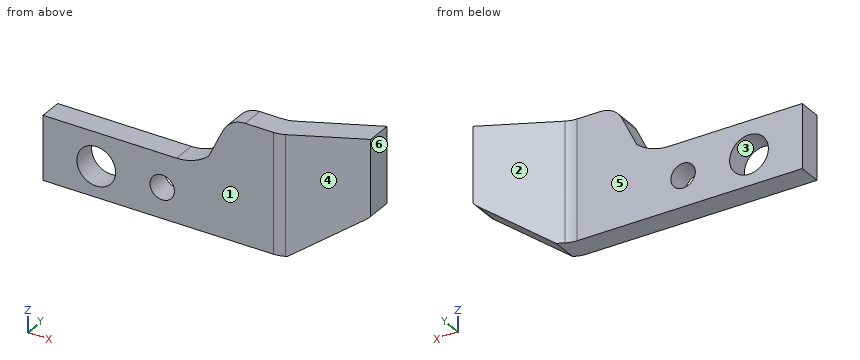
from build123d import *

# Parameters (mm, degrees)
SALIENTE_EXTRUIR1_DEPTH    = 100
CORTAR_EXTRUIR3_START      = -9.53
CORTAR_EXTRUIR3_DEPTH      = 27.53
CORTAR_EXTRUIR4_DEPTH      = 217.130875219
CORTAR_EXTRUIR4_DEPTH_BACK = 217.130875219
CROQUIS5_R                 = 6
CORTAR_EXTRUIR5_DEPTH      = 216.124741308
CORTAR_EXTRUIR5_DEPTH_BACK = 216.124741308
CROQUIS6_R                 = 5
SALIENTE_EXTRUIR5_START    = 15.13
CROQUIS12_R                = 8
CROQUIS12_R_2              = 6
SALIENTE_EXTRUIR5_DEPTH    = 15.13
CROQUIS14_R                = 10
CROQUIS14_R_2              = 6
SALIENTE_EXTRUIR6_DEPTH    = 14.13
REDONDEO1_R                = 10
CROQUIS15_R                = 129.913958972
CORTAR_EXTRUIR6_DEPTH      = 241.731126452
CORTAR_EXTRUIR7_DEPTH      = 241.731126452
CORTAR_EXTRUIR7_DEPTH_BACK = 241.731126452
CROQUIS16_R                = 167.818918699
CROQUIS16_W                = 152.833455663
CROQUIS16_H                = 57.32474986
CROQUIS17_R                = 7.94
CORTAR_EXTRUIR8_DEPTH      = 275.18730081


# Read off the part's stored shape, not the designer's step: Cortar-Extruir3
with BuildPart() as part:
    # Croquis1 → Saliente-Extruir1 (new body)
    with BuildSketch(Plane(origin=(0, 0, 0), x_dir=(-1, 0, 0), z_dir=(0, 0, 1))):
        Polygon((197, -18), (95.487511072, -18), (58.434265153, 0), (0, 0), (0, -9.53), (56.241982635, -9.53), (93.295228555, -27.53), (197, -27.53), align=None)
    extrude(amount=SALIENTE_EXTRUIR1_DEPTH)

    # Cortar-Extruir3 outline → Cortar-Extruir3 (cut)
    with BuildSketch(Plane.XZ.offset(-18).offset(CORTAR_EXTRUIR3_START)):
        with BuildLine():
            ThreePointArc((-55.249840127, 84.500440573), (-26.332291795, 96.782267833), (-21.152892526, 65.794500802))
            Line((-21.152892526, 65.794500802), (-64.625951049, 17.972279409))
            ThreePointArc((-64.625951049, 17.972279409), (-65.478127712, 17.140282818), (-66.423173576, 16.415498915))
            Line((-66.423173576, 16.415498915), (-90.606375863, 0.05961622))
            ThreePointArc((-90.606375863, 0.05961622), (-90.650882543, 0.029688544), (-90.695549093, 0))
            Line((-90.695549093, 0), (0, 0))
            Line((0, 0), (0, 100))
            Line((0, 100), (-197, 100))
            Line((-197, 100), (-197, 0))
            Line((-197, 0), (-190.011984345, 0))
            Line((-190.011984345, 0), (-190.011984345, 26.126101457))
            Line((-190.011984345, 26.126101457), (-135.299104154, 26.091319242))
            ThreePointArc((-135.299104154, 26.091319242), (-128.302319283, 27.350377114), (-122.187975643, 30.977363067))
            Line((-122.187975643, 30.977363067), (-116.240808663, 43.251828603))
            ThreePointArc((-116.240808663, 43.251828603), (-112.551713447, 47.365099857), (-107.241491018, 48.891521053))
            Line((-107.241491018, 48.891521053), (-89.308606426, 48.891521053))
            ThreePointArc((-89.308606426, 48.891521053), (-87.268864218, 49.101758455), (-85.31488803, 49.723630708))
            ThreePointArc((-85.31488803, 49.723630708), (-66.329070141, 63.694356674), (-55.249840127, 84.500440573))
        make_face()
    extrude(amount=CORTAR_EXTRUIR3_DEPTH, mode=Mode.SUBTRACT)

    # Croquis5 → Cortar-Extruir4 (cut, two sides: drawn at the far end of the back side and taken through both)
    with BuildSketch(Plane.XZ.offset(-CORTAR_EXTRUIR4_DEPTH_BACK)):
        with Locations(Location((-35.951954024, 79.247670643, 0), (0, 0, 270))):
            Circle(CROQUIS5_R)
    extrude(amount=CORTAR_EXTRUIR4_DEPTH + CORTAR_EXTRUIR4_DEPTH_BACK, mode=Mode.SUBTRACT)

    # Croquis6 → Cortar-Extruir5 (cut, two sides: drawn at the far end of the back side and taken through both)
    with BuildSketch(Plane.XZ.offset(-18).offset(-CORTAR_EXTRUIR5_DEPTH_BACK)):
        with Locations((-168.195527475, 12.5)):
            Circle(CROQUIS6_R)
        with Locations((-141.195527475, 12.5)):
            Circle(CROQUIS6_R)
    extrude(amount=CORTAR_EXTRUIR5_DEPTH + CORTAR_EXTRUIR5_DEPTH_BACK, mode=Mode.SUBTRACT)

    # Croquis12 → Saliente-Extruir5 (add)
    with BuildSketch(Plane.XZ.offset(SALIENTE_EXTRUIR5_START)):
        with Locations(Location((-35.951954024, 79.247670643, 0), (0, 0, 90))):
            Circle(CROQUIS12_R)
        with Locations(Location((-35.951954024, 79.247670643, 0), (0, 0, 270))):
            Circle(CROQUIS12_R_2, mode=Mode.SUBTRACT)
    extrude(amount=-SALIENTE_EXTRUIR5_DEPTH)

    # Croquis14 → Saliente-Extruir6 (add)
    with BuildSketch(Plane(origin=(0, -14.13, 0), x_dir=(-1, 0, 0), z_dir=(0, -1, 0))):
        with Locations(Location((35.951954024, -79.247670643, 0), (0, 0, 90))):
            Circle(CROQUIS14_R)
        with Locations(Location((35.951954024, -79.247670643, 0), (0, 0, 90))):
            Circle(CROQUIS14_R_2, mode=Mode.SUBTRACT)
    extrude(amount=-SALIENTE_EXTRUIR6_DEPTH)

    # Redondeo1
    redondeo1_edges = [part.edges().sort_by_distance(p)[0] for p in [
        (-95.487511072, 18, 24.445760526),
        (-58.434265153, 0, 50.31488072),
        (-93.295228555, 27.53, 24.445760526),
        (-56.241982635, 9.53, 54.230230798),
    ]]
    fillet(redondeo1_edges, radius=REDONDEO1_R)


with BuildPart() as body_2:
    # Simetría1: mirrored copy
    add(part.part.mirror(Plane(origin=(0, -82, 0), x_dir=(0, 0, 1), z_dir=(0, -1, 0))))


with BuildPart() as part_1:
    add(part.part)

    # Croquis15 → Cortar-Extruir6 (cut, through all)
    with BuildSketch(Plane(origin=(0, -82, 0), x_dir=(-1, 0, 0), z_dir=(0, -1, 0))):
        with Locations((137.546426993, -18.622395962)):
            Circle(CROQUIS15_R)
    extrude(amount=-CORTAR_EXTRUIR6_DEPTH, mode=Mode.SUBTRACT)


with BuildPart() as cortar_extruir7_tool:
    # Croquis16 → Cortar-Extruir7 (new, two sides: drawn at the far end of the back side and taken through both)
    with BuildSketch(Plane(origin=(0, -82, 0), x_dir=(-1, 0, 0), z_dir=(0, -1, 0)).offset(-CORTAR_EXTRUIR7_DEPTH_BACK)):
        with Locations((140.265045612, -47.269752677)):
            Circle(CROQUIS16_R)
        with Locations((141.042678881, -20.229146123)):
            Rectangle(CROQUIS16_W, CROQUIS16_H, mode=Mode.SUBTRACT)
    extrude(amount=CORTAR_EXTRUIR7_DEPTH + CORTAR_EXTRUIR7_DEPTH_BACK)


with BuildPart() as part_2:
    add(part_1.part)

    # Cortar-Extruir7: cut by cortar_extruir7_tool
    add(cortar_extruir7_tool.part, mode=Mode.SUBTRACT)


with BuildPart() as body_2_1:
    add(body_2.part)

    # Cortar-Extruir7: cut by cortar_extruir7_tool
    add(cortar_extruir7_tool.part, mode=Mode.SUBTRACT)

    # Croquis17 → Cortar-Extruir8 (cut, through all)
    with BuildSketch(Plane(origin=(0, 0, 0), x_dir=(1, 0, 0), z_dir=(0, 1, 0))):
        with Locations(Location((-168.195527475, -12.5, 0), (0, 0, 270))):
            Circle(CROQUIS17_R)
    extrude(amount=-CORTAR_EXTRUIR8_DEPTH, mode=Mode.SUBTRACT)


solid = body_2_1.part
Read the model definition and answer for the solid it produces. Units are mm, in the model's axes. Face numbers are marked on the shaded views. A direction names the side the tool comes from. Round coordinates to 2 decimals unless told otherwise and drop trailing zeros. Write each loop counter-clockwise with the first axis right and the second up, starting at its lowest first coordinate (ties: lowest second). Pieces come first, ordered by that corner, then holes. Notation, with made-up numbers: M 58,-11 L 88,-11 A29 cw 88,9 Z; hole C 87,26.25 d6. An arc over 180 degrees is marked long. Use a Markdown table: item, result.
1) Straight lines are drawn through the part: line 1 along X through (y, z) = (-187.25, 12.5); line 2 along X through (y, z) = (-184.5, 12.5); line 3 along Y through (x, z) = (-115, 45). For each, find the intervals that lie inside material, in ascending order. Write a range as [from, to].
Answers follow:
| item | result |
|---|---|
| line 1 | x = [-190.01, -176.14], [-160.26, -146.2], [-136.2, -84.48] |
| line 2 | x = [-190.01, -176.14], [-160.26, -146.2], [-136.2, -78.82] |
| line 3 | y = [-191.53, -182] |
2) The part is cut by section B-B (z = 12.5). Write down the section's boundary in (x, y).
Answers follow:
| item | result |
|---|---|
| outline | M -190.01,-191.53 L -176.14,-191.53 L -176.14,-182 L -190.01,-182 Z; M -160.26,-191.53 L -146.2,-191.53 L -146.2,-182 L -160.26,-182 Z; M -136.2,-191.53 L -95.6,-191.53 A10 ccw -91.23,-190.52 L -72.21,-181.29 L -72.21,-170.69 L -93.42,-180.99 A10 cw -97.79,-182 L -136.2,-182 Z |
3) The part is cut by section D-D (y = -176). Write down the section's boundary in (x, z), plus the area to 3 significant figures.
Answers follow:
| item | result |
|---|---|
| outline | M -83.14,5.11 L -66.42,16.42 A10 ccw -64.63,17.97 L -64.63,48.89 L -83.14,48.89 Z |
| area | 694 mm2 |
4) The part is cut by section A-A (x = -167). Write down the section's boundary in (y, z), plus the area to 3 significant figures.
Answers follow:
| item | result |
|---|---|
| outline | M -191.53,0 L -182,0 L -182,4.65 L -191.53,4.65 Z; M -191.53,20.35 L -182,20.35 L -182,26.11 L -191.53,26.11 Z |
| area | 99.2 mm2 |
5) A tool of negligible diameter and unlimited length cuts with its end or side. For the marked faces 5 and 6, from which of +Z, -Z, +X, -X, +Y, -Y can it reach the whole face along a straight path? Write none if from no direction.
Answers follow:
| item | result |
|---|---|
| face 5 | +Z, -Z, -X, +Y |
| face 6 | +Z, -Z, +X, +Y, -Y |
6) The part is cut by section C-C (z = 29). Write down the section's boundary in (x, y), plus the area to 3 significant figures.
Answers follow:
| item | result |
|---|---|
| outline | M -124.9,-191.53 L -95.6,-191.53 A10 ccw -91.23,-190.52 L -64.63,-177.6 L -64.63,-167.01 L -93.42,-180.99 A10 cw -97.79,-182 L -124.9,-182 Z |
| area | 606 mm2 |
7) For a pull along X with two mould halves and no side action, classify the marked faces 1, 2, 3 and 4 as pulls with the +X half, pulls with the -X half, needs draft (parallel to the pull), parting line crosses it, or undercut.
Answers follow:
| item | result |
|---|---|
| face 1 | needs draft |
| face 2 | pulls with the -X half |
| face 3 | undercut |
| face 4 | pulls with the +X half |
8) Flat-ended cylindrical pins translate along their axes: pin 1 (3 mm diameter, centred on y = -175, z = 9, fed in from +X); pin 2 (12 mm diameter, centred on x = -109.5, z = 14.5, fed in from +Y); pin 3 (3 mm diameter, centred on x = -84, y = -188, fed in from +Z); pin 4 (4 mm diameter, centred on y = -175, z = 24.5, fed in from -X). Find the tip coordinate at first contact, or state that the pin passes through.
Answers follow:
| item | result |
|---|---|
| pin 1 | stops at x = -75.17 |
| pin 2 | stops at y = -182 |
| pin 3 | stops at z = 48.89 |
| pin 4 | stops at x = -85.19 |
